Could you check a few things on this drawing? It's one solid part, dimensions in mm from its lowest x, y, z. A direction names the side the tool comes from. Give positions to 0.01 mm unless a question says otherwise; leave off trailing zeros. Write each loop counter-clockwise with the first axis right and the second up, starting at its lowest first coordinate (ties: lowest second). Pieces come first, ordered by that corner, then holes. Notation, with made-up numbers: (37.25, 82.5) -> (67.25, 82.5) arc R21 ccw to (67.25, 99.5) -> close; hole circle Ø11 at (49, -23). An arc over 180 degrees is marked (long way). Answer as CSV lines item,"result". Start each with the question number.
1. If we section it at A-A on y = 35.5: Write out the boundary of the cut face in (x, z).
2. I'm going to push flat-ended pins straight in: P1, Ø3, axis at y = 30, z = 64.5, coming from the -X side; P2, Ø17.5, axis at x = 39.5, y = 44, coming from the +Z side; P3, Ø1, axis at y = 27, z = 51.5, coming from the -X side; P4, Ø3, axis at y = 31, z = 54, coming from the +X side. Where does each tip first touch, or does it pass through?
3. If we section it at B-B on x = 33.5: Write out the boundary of the cut face in (y, z).
4. If we section it at C-C on z = 37: Write out the boundary of the cut face in (x, y).
5. On a 3-axis mill with a long thin cutter (end or side, diameter ignored), from which of +Z, -Z, +X, -X, +Y, -Y can I reach the whole of each face in a straight line? I mean the marked faces 1, 2, 3, 4 and 5. Say none if no direction works.
6. I need wall thicknesses on line 1 (Z direction, x = 12, y = 11); line 2 (X direction, y = 29.5, z = 36); line 3 (Z direction, x = 41.5, y = 52). Which ranges of each line are inside material? Lowest first, please. Write a range as [from, to].
7. If we section it at D-D on z = 82: Write out the boundary of the cut face in (x, y).
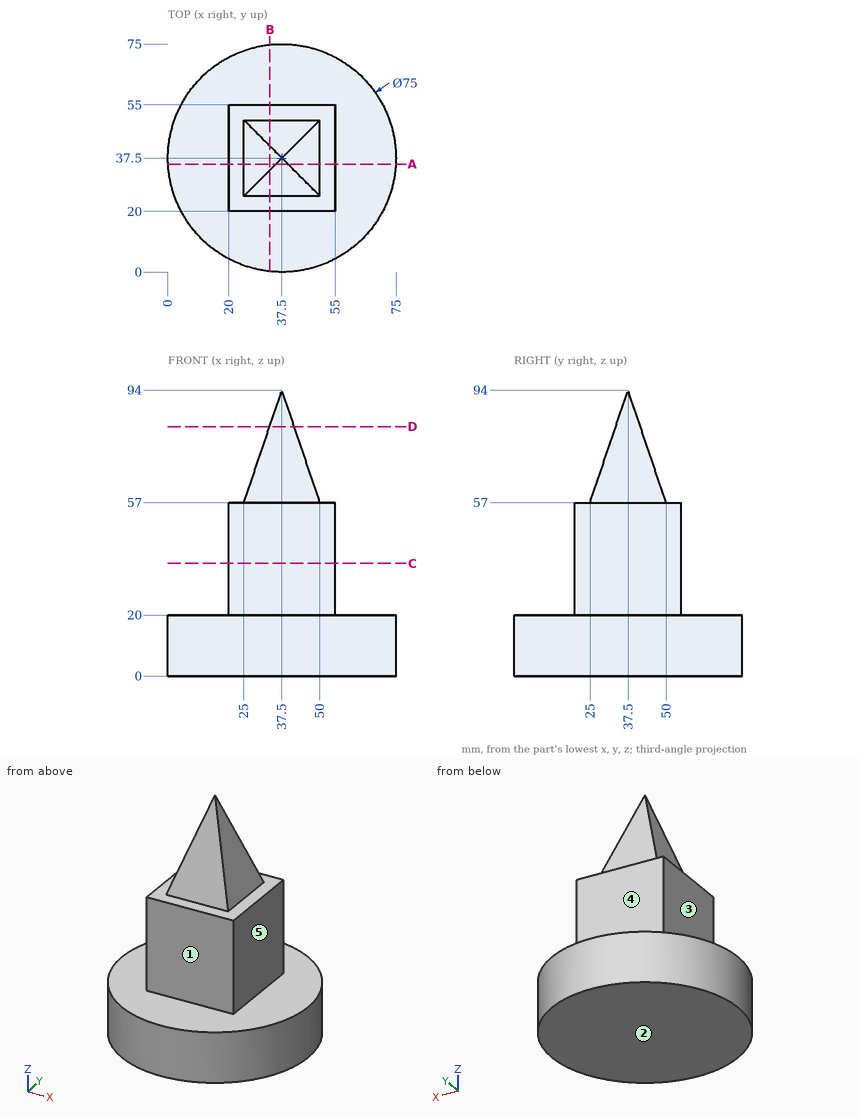
Computed values:
1,outline,"(0.05, 0) -> (74.95, 0) -> (74.95, 20) -> (55, 20) -> (55, 57) -> (50, 57) -> (39.5, 88.08) -> (35.5, 88.08) -> (25, 57) -> (20, 57) -> (20, 20) -> (0.05, 20) -> close"
2,P1,"stops at x = 27.03"
2,P2,"stops at z = 94"
2,P3,"stops at x = 20"
2,P4,"stops at x = 55"
3,outline,"(0.21, 0) -> (74.79, 0) -> (74.79, 20) -> (55, 20) -> (55, 57) -> (50, 57) -> (41.5, 82.16) -> (33.5, 82.16) -> (25, 57) -> (20, 57) -> (20, 20) -> (0.21, 20) -> close"
4,outline,"(20, 20) -> (55, 20) -> (55, 55) -> (20, 55) -> close"
5,face 1,"+Z, +X, -X, -Y"
5,face 2,"-Z, +X, -X, +Y, -Y"
5,face 3,"+Z, -X, +Y, -Y"
5,face 4,"+Z, +X, -X, +Y"
5,face 5,"+Z, +X, +Y, -Y"
6,line 1,"z = [0, 20]"
6,line 2,"x = [20, 55]"
6,line 3,"z = [0, 57]"
7,outline,"(33.45, 33.45) -> (41.55, 33.45) -> (41.55, 41.55) -> (33.45, 41.55) -> close"
